For this review, use the dimensioned drawing (mm, ordinates from the lowest corner) and the shaded views. A direction names the side the tool comes from. Coordinates: 2 decimals unless noted, no trailing zeros. Write each loop counter-clockwise with the first axis right and the second up, starting at its lowest first coordinate (ties: lowest second). Pieces come first, ordered by that corner, then holes.
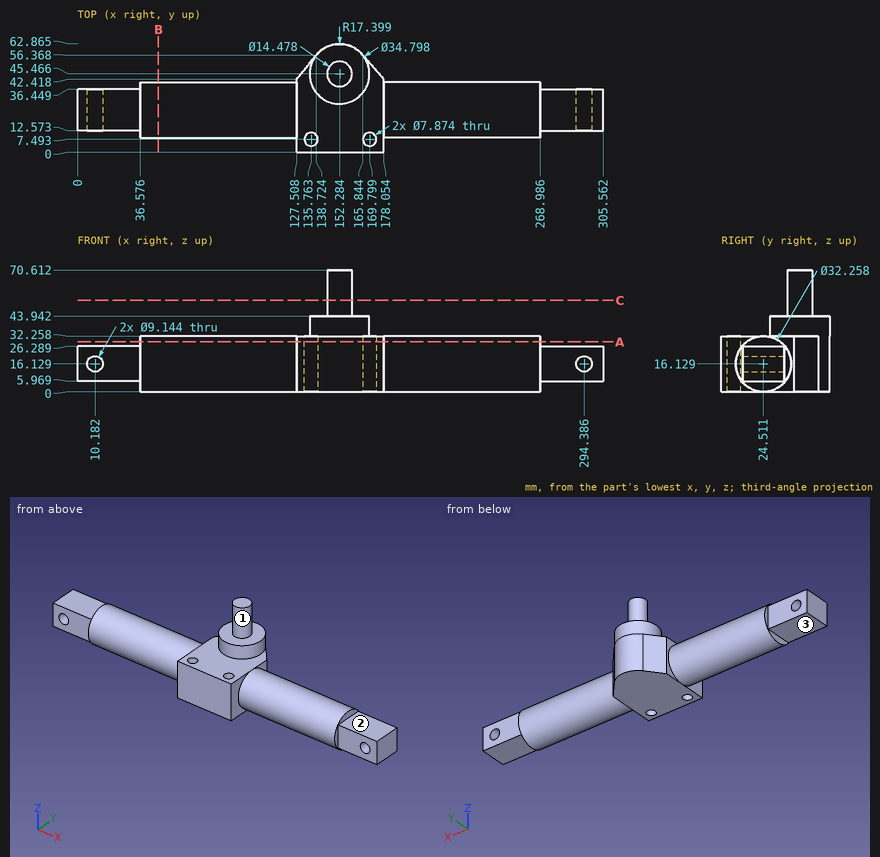
Item 1: Take a section at C-C, the plane z = 53. Write out the cut boundary in (x, y).
Solved:
outline: circle Ø14.48 at (152.28, 45.47)
Item 2: Take a section at A-A, the plane z = 29. Write out the cut boundary in (x, y), plus the area to 3 significant figures.
Solved:
outline: (36.58, 14.79) - (127.51, 14.79) - (127.51, 0) - (178.05, 0) - (178.05, 14.79) - (268.99, 14.79) - (268.99, 34.23) - (178.05, 34.23) - (178.05, 42.42) - (165.84, 56.37) arc R17.4 ccw to (138.72, 56.37) - (127.51, 42.42) - (127.51, 34.23) - (36.58, 34.23) - close; hole circle Ø7.87 at (135.76, 7.49); hole circle Ø7.87 at (169.8, 7.49)
area: 6,250 mm2
Item 3: To check wall thickness, follow line 1 along X through (y, z) = (31, 18) (1 decimal); line 2 along Z through (x, y) = (176, 39); line 3 along X through (y, z) = (37, 10.5). State the ranges of each line that lie inside material, in increasing order.
Solved:
line 1: x = 0 to 6, 14.4 to 290.2, 298.6 to 305.6
line 2: z = 0 to 32.26
line 3: x = 36.58 to 268.99
Item 4: Machinability: for the marked faces 1, 2 and 3, which of the approach directions +Z, -Z, +X, -X, +Y, -Y give a long, thin tool a straight path to every point of the face, cutting with its end or side? Answer none if there is none.
Solved:
face 1: +Z
face 2: +Z, +X, +Y, -Y
face 3: -Z, -X, +Y, -Y
Item 5: For pin 1 (6 mm diameter, centred on x = 286.5, z = 12, fed in from -Y); pin 2 (8 mm diameter, centred on x = 10.18, z = 16.13, fed in from +Y); pin 3 (1.5 mm diameter, centred on x = 250.5, y = 9.5, fed in from -Z) (1 decimal); pin 4 (14.5 mm diameter, centred on x = 294.386, z = 16.129, fed in from +Y), all flat-tipped, find the tip position at first contact; note any pin that passes through.
Solved:
pin 1: stops at y = 12.57
pin 2: passes through
pin 3: stops at z = 8.6
pin 4: stops at y = 36.45
Item 6: Take a section at B-B, the plane x = 47. Write out the cut boundary in (y, z), plus the area to 3 significant figures.
Solved:
outline: circle Ø32.26 at (24.51, 16.13)
area: 817 mm2
